Read the model definition and answer for the solid it produces. Units are mm, in the model's axes. Face numbers are marked on the shaded views. A direction names the side the tool comes from. Coordinates: 2 decimals unless noted, no trailing zeros. Loops run counter-clockwise (first coordinate to the right, second up) from the corner with the lowest first, then second, coordinate; pieces in that order, holes last. Notation, with made-up numbers: (-39.75, 20) - (-31.75, 20) arc R27 cw to (-31.75, 37) - close; hole circle Ø9 at (-36.75, 28.5). An arc over 180 degrees is marked (long way). Use CSV: the item, a comma, the result in double quotes.
```python
from build123d import *

# Parameters (mm, degrees)
SKETCH1_R           = 8.44
BOSS_EXTRUDE1_DEPTH = 24
SKETCH2_W           = 9.525
SKETCH2_H           = 9.525
CUT_EXTRUDE1_DEPTH  = 11.44
SKETCH3_R           = 4.5
CUT_EXTRUDE2_DEPTH  = 18.32688085
CUT_EXTRUDE3_DEPTH  = 8
FILLET1_R           = 1


with BuildPart() as part:
    # Sketch1 → Boss-Extrude1 (new body)
    with BuildSketch(Plane(origin=(0, 0, 0), x_dir=(1, 0, 0), z_dir=(0, 1, 0))):
        with Locations(Location((0, 0, 0), (0, 0, 270))):
            Circle(SKETCH1_R)
    extrude(amount=BOSS_EXTRUDE1_DEPTH)

    # Sketch2 → Cut-Extrude1 (cut)
    with BuildSketch(Plane(origin=(0, 24, 0), x_dir=(1, 0, 0), z_dir=(0, 1, 0))):
        Rectangle(SKETCH2_W, SKETCH2_H)
    extrude(amount=-CUT_EXTRUDE1_DEPTH, mode=Mode.SUBTRACT)

    # Sketch3 → Cut-Extrude2 (cut, through all)
    with BuildSketch(Plane(origin=(0, 12.56, 0), x_dir=(1, 0, 0), z_dir=(0, 1, 0))):
        with Locations(Location((0, 0, 0), (0, 0, 270))):
            Circle(SKETCH3_R)
    extrude(amount=-CUT_EXTRUDE2_DEPTH, mode=Mode.SUBTRACT)

    # Sketch4 → Cut-Extrude3 (cut)
    with BuildSketch(Plane.XZ):
        Polygon((-3.207902433, 5.55625), (-6.415804866, 0), (-3.207902433, -5.55625), (3.207902433, -5.55625), (6.415804866, 0), (3.207902433, 5.55625), align=None)
    extrude(amount=-CUT_EXTRUDE3_DEPTH, mode=Mode.SUBTRACT)

    # Sketch5 → Cut-Revolve1 (revolve, cut)
    with BuildSketch(Plane(origin=(0, 0, 0), x_dir=(0, 0, -1), z_dir=(1, 0, 0))):
        with BuildLine():
            Line((-6.55625, 0), (-5.55625, 0))
            Line((-5.55625, 0), (-5.55625, 1))
            ThreePointArc((-5.55625, 1), (-5.849143219, 0.292893219), (-6.55625, 0))
        make_face()
        with BuildLine():
            Line((-6.7625, 24), (-4.7625, 24))
            Line((-4.7625, 24), (-4.7625, 22))
            ThreePointArc((-4.7625, 22), (-5.348286438, 23.414213562), (-6.7625, 24))
        make_face()
    revolve(axis=Axis((0, 24, 0), (0, -1, 0)), mode=Mode.SUBTRACT)

    # Fillet1
    fillet1_edges = [part.edges().sort_by_distance(p)[0] for p in [
        (0, 0, -8.44),
        (0, 24, -8.44),
    ]]
    fillet(fillet1_edges, radius=FILLET1_R)


solid = part.part
```
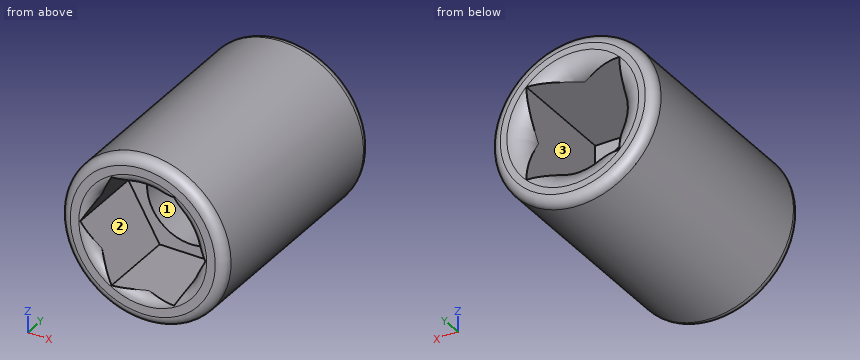
Q1. Given P1, Ø8, axis at x = -0.5, z = 1, coming from the +Y side; P2, Ø3.5, axis at x = 2.5, z = -2, coming from the -Y side; P3, Ø3, axis at y = 20, z = -6.5, coming from the -X side, each flat-ended and moving along its own axis, determine where each tip first touches the part or whether it passes through.
Reported:
P1,"stops at y = 23.13"
P2,"stops at y = 8"
P3,"stops at x = -6.8"
Q2. The part is cut by section C-C on y = 11.75. Determine the outline of the cut face in (x, z).
Reported:
outline,"circle Ø16.88 at (0, 0); hole circle Ø9 at (0, 0)"
Q3. The part is cut by section A-A on x = 0. Determine the outline of the cut face in (y, z).
Reported:
outline,"(0, -7.44) arc R1 ccw to (1, -8.44) - (23, -8.44) arc R1 ccw to (24, -7.44) - (24, -6.76) arc R2 ccw to (22, -4.76) - (12.56, -4.76) - (12.56, -4.5) - (8, -4.5) - (8, -5.56) - (1, -5.56) arc R1 ccw to (0, -6.56) - close; (0, 6.56) arc R1 ccw to (1, 5.56) - (8, 5.56) - (8, 4.5) - (12.56, 4.5) - (12.56, 4.76) - (22, 4.76) arc R2 ccw to (24, 6.76) - (24, 7.44) arc R1 ccw to (23, 8.44) - (1, 8.44) arc R1 ccw to (0, 7.44) - close"
Q4. A tool of negligible diameter and unlimited length cuts with its end or side. For the marked faces 1, 2 and 3, from which of +Z, -Z, +X, -X, +Y, -Y can it reach the whole face along a straight path? Write none if from no direction.
Reported:
face 1,"+Y, -Y"
face 2,"-Y"
face 3,"+Y"
Q5. Find the intervals of material crossed by probe 1 along X at (y, z) = (10.4, 0); probe 2 along X at (y, z) = (15, 0); probe 3 along Y at (x, z) = (1.75, 4.25), in increasing order. Write a range as [from, to].
Reported:
probe 1,"x = [-8.44, -4.5], [4.5, 8.44]"
probe 2,"x = [-8.44, -4.76], [4.76, 8.44]"
probe 3,"y = [8, 12.56]"
Q6. The part is cut by section B-B on y = 14.75. Determine the outline of the cut face in (x, z), and give its area (3 significant figures).
Reported:
outline,"circle Ø16.88 at (0, 0); hole (-4.76, -4.76) - (4.76, -4.76) - (4.76, 4.76) - (-4.76, 4.76) - close"
area,"133 mm²"
